```python
from build123d import *

# Parameters (mm, degrees)
SKETCH1_W           = 139.7
SKETCH1_H           = 76.2
BOSS_EXTRUDE1_DEPTH = 31.75
SKETCH2_W           = 128.27
SKETCH2_H           = 63.545947231
CUT_EXTRUDE1_DEPTH  = 25.4
SKETCH3_W           = 10.16
SKETCH3_H           = 10.16
BOSS_EXTRUDE3_DEPTH = 12.7
SKETCH4_R           = 2.032
CUT_EXTRUDE2_DEPTH  = 82.814026915
SKETCH5_R           = 3.937
CUT_EXTRUDE3_DEPTH  = 2.286
SKETCH7_R           = 2.54
SKETCH7_R_2         = 1.6002
BOSS_EXTRUDE5_DEPTH = 3.175
BOSS_EXTRUDE6_DEPTH = 3.175
SKETCH9_W           = 3.175
SKETCH9_H           = 38.1
BOSS_EXTRUDE7_DEPTH = 28.575
SKETCH10_R          = 5.5499
CUT_EXTRUDE4_DEPTH  = 3.175
SKETCH11_R          = 9.525
CUT_EXTRUDE5_DEPTH  = 3.175
SKETCH12_R          = 12.7
CUT_EXTRUDE6_DEPTH  = 3.175


with BuildPart() as part:
    # Sketch1 → Boss-Extrude1 (new body)
    with BuildSketch(Plane(origin=(0, 0, 0), x_dir=(1, 0, 0), z_dir=(0, 1, 0))):
        Rectangle(SKETCH1_W, SKETCH1_H)
    extrude(amount=BOSS_EXTRUDE1_DEPTH)

    # Sketch2 → Cut-Extrude1 (cut)
    with BuildSketch(Plane(origin=(0, 31.75, 0), x_dir=(1, 0, 0), z_dir=(0, 1, 0))):
        with Locations((5.715, 6.372973615)):
            Rectangle(SKETCH2_W, SKETCH2_H)
    extrude(amount=-CUT_EXTRUDE1_DEPTH, mode=Mode.SUBTRACT)

    # Sketch3 → Boss-Extrude3 (add)
    with BuildSketch(Plane(origin=(0, 6.35, 0), x_dir=(1, 0, 0), z_dir=(0, 1, 0))):
        with Locations((-53.34, -20.32)):
            Rectangle(SKETCH3_W, SKETCH3_H)
    extrude(amount=BOSS_EXTRUDE3_DEPTH)

    # Sketch4 → Cut-Extrude2 (cut, through all)
    with BuildSketch(Plane(origin=(0, 19.05, 0), x_dir=(1, 0, 0), z_dir=(0, 1, 0))):
        with Locations(Location((-53.34, -20.32, 0), (0, 0, 270))):
            Circle(SKETCH4_R)
    extrude(amount=-CUT_EXTRUDE2_DEPTH, mode=Mode.SUBTRACT)

    # Sketch5 → Cut-Extrude3 (cut)
    with BuildSketch(Plane(origin=(0, 19.05, 0), x_dir=(1, 0, 0), z_dir=(0, 1, 0))):
        with Locations(Location((-53.34, -20.32, 0), (0, 0, 270))):
            Circle(SKETCH5_R)
    extrude(amount=-CUT_EXTRUDE3_DEPTH, mode=Mode.SUBTRACT)

    # Sketch7 → Boss-Extrude5 (add)
    # profile 1 of 6: a face of its own
    with BuildSketch(Plane(origin=(0, 6.35, 0), x_dir=(1, 0, 0), z_dir=(0, 1, 0))):
        with Locations(Location((-30.48, 30.48, 0), (0, 0, 90))):
            Circle(SKETCH7_R)
        with Locations(Location((-30.48, 30.48, 0), (0, 0, 270))):
            Circle(SKETCH7_R_2, mode=Mode.SUBTRACT)
    # profile 2 of 6: a face of its own
    with BuildSketch(Plane(origin=(0, 6.35, 0), x_dir=(1, 0, 0), z_dir=(0, 1, 0))):
        with Locations(Location((-24.13, -17.78, 0), (0, 0, 90))):
            Circle(SKETCH7_R)
        with Locations(Location((-24.13, -17.78, 0), (0, 0, 270))):
            Circle(SKETCH7_R_2, mode=Mode.SUBTRACT)
    # profile 3 of 6: a face of its own
    with BuildSketch(Plane(origin=(0, 6.35, 0), x_dir=(1, 0, 0), z_dir=(0, 1, 0))):
        with Locations(Location((0, 25.4, 0), (0, 0, 90))):
            Circle(SKETCH7_R)
        with Locations(Location((0, 25.4, 0), (0, 0, 270))):
            Circle(SKETCH7_R_2, mode=Mode.SUBTRACT)
    # profile 4 of 6: a face of its own
    with BuildSketch(Plane(origin=(0, 6.35, 0), x_dir=(1, 0, 0), z_dir=(0, 1, 0))):
        with Locations(Location((0, -2.54, 0), (0, 0, 90))):
            Circle(SKETCH7_R)
        with Locations(Location((0, -2.54, 0), (0, 0, 270))):
            Circle(SKETCH7_R_2, mode=Mode.SUBTRACT)
    # profile 5 of 6: a face of its own
    with BuildSketch(Plane(origin=(0, 6.35, 0), x_dir=(1, 0, 0), z_dir=(0, 1, 0))):
        with Locations(Location((50.8, -17.78, 0), (0, 0, 90))):
            Circle(SKETCH7_R)
        with Locations(Location((50.8, -17.78, 0), (0, 0, 270))):
            Circle(SKETCH7_R_2, mode=Mode.SUBTRACT)
    # profile 6 of 6: a face of its own
    with BuildSketch(Plane(origin=(0, 6.35, 0), x_dir=(1, 0, 0), z_dir=(0, 1, 0))):
        with Locations(Location((52.07, 30.48, 0), (0, 0, 90))):
            Circle(SKETCH7_R)
        with Locations(Location((52.07, 30.48, 0), (0, 0, 270))):
            Circle(SKETCH7_R_2, mode=Mode.SUBTRACT)
    extrude(amount=BOSS_EXTRUDE5_DEPTH)

    # Sketch8 → Boss-Extrude6 (add)
    with BuildSketch(Plane.XZ):
        Polygon((-69.85, 38.1), (-69.85, 76.2), (-12.7, 76.2), (25.4, 38.1), align=None)
    extrude(amount=-BOSS_EXTRUDE6_DEPTH)

    # Sketch9 → Boss-Extrude7 (add)
    with BuildSketch(Plane(origin=(0, 3.175, 0), x_dir=(1, 0, 0), z_dir=(0, 1, 0))):
        with Locations((-68.2625, -57.15)):
            Rectangle(SKETCH9_W, SKETCH9_H)
        Polygon((-8.8265, -72.3265), (-11.07156403, -74.57156403), (-11.07156403, -38.1), (-8.8265, -38.1), align=None)
        with Locations((-54.864, -57.15)):
            Rectangle(SKETCH9_W, SKETCH9_H)
    extrude(amount=BOSS_EXTRUDE7_DEPTH)

    # Sketch10 → Cut-Extrude4 (cut)
    with BuildSketch(Plane.ZY.offset(69.85)):
        with Locations((57.15, 15.875)):
            Circle(SKETCH10_R)
    extrude(amount=-CUT_EXTRUDE4_DEPTH, mode=Mode.SUBTRACT)

    # Sketch11 → Cut-Extrude5 (cut)
    with BuildSketch(Plane.ZY.offset(56.4515)):
        with Locations((57.15, 15.875)):
            Circle(SKETCH11_R)
    extrude(amount=-CUT_EXTRUDE5_DEPTH, mode=Mode.SUBTRACT)

    # Sketch12 → Cut-Extrude6 (cut)
    with BuildSketch(Plane.ZY.offset(11.07156403)):
        with Locations(Location((57.15, 15.875, 0), (0, 0, 270))):
            Circle(SKETCH12_R)
    extrude(amount=-CUT_EXTRUDE6_DEPTH, mode=Mode.SUBTRACT)


solid = part.part
```
Check sheet for the modelled part. Datum: model origin and axes. Units: mm. A direction names the side the tool comes from. Round coordinates to 2 decimals unless told otherwise and drop trailing zeros. Order: outer loops, then holes, each group sorted by start corner. A loop starts at its lowest first (then second) coordinate and runs counter-clockwise, first axis right, second up. Notation, with made-up numbers: (14, 62.5) -> (60, 62.5) arc R10 cw to (60, 66.5) -> close; hole circle Ø6 at (88, 19.5). An arc over 180 degrees is marked (long way). Use CSV: the item, a comma, the result in double quotes.
(1) Cross-section at A-A (x = -40). Record the boundary of the cut face in (y, z) (3 decimals).
Worked out:
outline,"(0, -38.1) -> (6.35, -38.1) -> (6.35, 25.4) -> (31.75, 25.4) -> (31.75, 38.1) -> (3.175, 38.1) -> (3.175, 76.2) -> (0, 76.2) -> close"
(2) Material ranges on line 1 along X through (y, z) = (8, -25); line 2 along Z through (x, y) = (-31, 17); line 3 along Z through (x, y) = (-63, 13), recorded low to high. Write a range as from..to.
Worked out:
line 1,"-69.85..-58.42, -2.51..-1.55, 1.55..2.51"
line 2,"25.4..38.1"
line 3,"-38.1..38.1"
(3) Cross-section at C-C (x = 0). Record the boundary of the cut face in (y, z) (3 decimals), and give its area (3 significant figures).
Worked out:
outline,"(0, -38.1) -> (6.35, -38.1) -> (6.35, -27.94) -> (9.525, -27.94) -> (9.525, -27) -> (6.35, -27) -> (6.35, -23.8) -> (9.525, -23.8) -> (9.525, -22.86) -> (6.35, -22.86) -> (6.35, 0) -> (9.525, 0) -> (9.525, 0.94) -> (6.35, 0.94) -> (6.35, 4.14) -> (9.525, 4.14) -> (9.525, 5.08) -> (6.35, 5.08) -> (6.35, 25.4) -> (31.75, 25.4) -> (31.75, 38.1) -> (3.175, 38.1) -> (3.175, 63.5) -> (0, 63.5) -> close"
area,"899 mm²"
(4) Cross-section at D-D (z = 2.54). Record the boundary of the cut face in (x, y) (3 decimals).
Worked out:
outline,"(-69.85, 0) -> (69.85, 0) -> (69.85, 6.35) -> (2.54, 6.35) -> (2.54, 9.525) -> (1.6, 9.525) -> (1.6, 6.35) -> (-1.6, 6.35) -> (-1.6, 9.525) -> (-2.54, 9.525) -> (-2.54, 6.35) -> (-58.42, 6.35) -> (-58.42, 31.75) -> (-69.85, 31.75) -> close"
(5) Tool access check on faces 4 (the face through (49.24, 7.92, 17.43)), 5 (the face through (-9.965, 18.628, 44.752)), 6 (the face through (-53.276, 20, 66)), 7 (the face through (-53, 13, 15.24)). Record the directions out of +Z, -Z, +X, -X, +Y, -Y that give a thin tool (end or side, any length) a straight path to the whole face; none if there is none.
Worked out:
face 4,"+Y"
face 5,"+X"
face 6,"+Z, +Y"
face 7,"-Z, +X, +Y"
(6) Depth check by flat-ended pin: pin 1 (2 mm diameter, centred on x = -13.5, z = -23, fed in from +Y); pin 2 (7.5 mm diameter, centred on y = 18.5, z = 1, fed in from +X); pin 3 (19 mm diameter, centred on x = 7.5, z = 1.5, fed in from +Y) (3 decimals). Enter the tip coordinate at first touch or a pass-through.
Worked out:
pin 1,"y = 6.35"
pin 2,"x = -58.42"
pin 3,"y = 9.525"
(7) Draft check along X on faces 1 (the face through (-68.285, 13.749, 62.277)), 2 (the face through (-49.437, 17.923, 19.807)), 3 (the face through (-2.2, 2.9, 65.7)). Enter one of: pulls with the +X half, pulls with the -X half, needs draft (parallel to the pull), parting line crosses it, or undercut.
Worked out:
face 1,"needs draft"
face 2,"undercut"
face 3,"pulls with the +X half"
